```python
from build123d import *

# Parameters (mm, degrees)
EXTRUDE_1_DEPTH     = 50
SKETCH_4_W          = 44
SKETCH_4_H          = 13
CUT_EXTRUDE_2_DEPTH = 20
CUT_EXTRUDE_3_DEPTH = 88.252507127
SKETCH_6_R          = 11.05
SKETCH_6_R_2        = 1.6
CUT_EXTRUDE_4_DEPTH = 88.183714076


with BuildPart() as part:
    # 草图1 → 凸台-拉伸1 (new body)
    with BuildSketch(Plane(origin=(0, 0, 0), x_dir=(0, 0, -1), z_dir=(1, 0, 0))):
        Polygon((3, 0), (0, 0), (0, -51), (53, -51), (53, -48), (16, -48), (3, -28), align=None)
    extrude(amount=EXTRUDE_1_DEPTH)

    # 草图4 → 切除-拉伸2 (cut)
    with BuildSketch(Plane(origin=(0, -48, 0), x_dir=(1, 0, 0), z_dir=(0, 1, 0))):
        with Locations((25, 9.5)):
            Rectangle(SKETCH_4_W, SKETCH_4_H)
    extrude(amount=CUT_EXTRUDE_2_DEPTH, mode=Mode.SUBTRACT)

    # 草图5 → 切除-拉伸3 (cut, through all)
    with BuildSketch(Plane(origin=(0, -48, 0), x_dir=(1, 0, 0), z_dir=(0, 1, 0))):
        with BuildLine():
            Line((12.1, 42), (12.1, 12))
            ThreePointArc((12.1, 12), (10, 9.9), (7.9, 12))
            Line((7.9, 12), (7.9, 42))
            ThreePointArc((7.9, 42), (10, 44.1), (12.1, 42))
        make_face()
        with BuildLine():
            Line((37.9, 42), (37.9, 12))
            ThreePointArc((37.9, 12), (40, 9.9), (42.1, 12))
            Line((42.1, 12), (42.1, 42))
            ThreePointArc((42.1, 42), (40, 44.1), (37.9, 42))
        make_face()
        Polygon((50, 53), (45, 53), (50, 48), align=None)
        Polygon((5, 53), (0, 48), (0, 53), align=None)
    extrude(amount=-CUT_EXTRUDE_3_DEPTH, mode=Mode.SUBTRACT)

    # 草图6 → 切除-拉伸4 (cut, through all)
    with BuildSketch(Plane(origin=(0, 0, -3), x_dir=(-1, 0, 0), z_dir=(0, 0, -1))):
        with Locations(Location((-25, -21, 0), (0, 0, 90))):
            Circle(SKETCH_6_R)
        with Locations(Location((-40.5, -5.5, 0), (0, 0, 90))):
            Circle(SKETCH_6_R_2)
        with Locations(Location((-9.5, -5.5, 0), (0, 0, 90))):
            Circle(SKETCH_6_R_2)
        with Locations(Location((-9.5, -36.5, 0), (0, 0, 90))):
            Circle(SKETCH_6_R_2)
        with Locations(Location((-40.5, -36.5, 0), (0, 0, 90))):
            Circle(SKETCH_6_R_2)
        Polygon((-50, 0), (-50, -5), (-45, 0), align=None)
        Polygon((0, -5), (-5, 0), (0, 0), align=None)
    extrude(amount=-CUT_EXTRUDE_4_DEPTH, mode=Mode.SUBTRACT)


solid = part.part
```
The model under review builds one solid part; all positions refer to its coordinate system, in mm. A direction names the side the tool comes from. Round coordinates to 2 decimals unless told otherwise and drop trailing zeros. Write each loop counter-clockwise with the first axis right and the second up, starting at its lowest first coordinate (ties: lowest second). Pieces come first, ordered by that corner, then holes. Notation, with made-up numbers: (-3, -14.5) - (11, -14.5) arc R25 cw to (11, 14.5) - close; hole circle Ø9 at (-20, 77.25). An arc over 180 degrees is marked (long way). Use one line per item in the form item = value.
Q1. Insertion check: pin 1 Ø5 at (x, y) = (40.5, -36.5) entering from -Z; pin 2 Ø4 at (x, z) = (41, -6.5) entering from +Y; pin 3 Ø14.5 at (y, z) = (-34.5, -7.5) entering from +X. Each pin has a flat end and moves straight along its axis. Give the tip position at first contact, or say it passes through.
Answer key:
pin_1 = -3
pin_2 = -48
pin_3 = 50
Q2. Consider section C-C (z = -34.5). State the section outline as (x, y) points.
Answer key:
outline = (0, -51) - (7.9, -51) - (7.9, -48) - (0, -48) - close; (12.1, -51) - (37.9, -51) - (37.9, -48) - (12.1, -48) - close; (42.1, -51) - (50, -51) - (50, -48) - (42.1, -48) - close
Q3. Tool access review of faces 5 (the flat face through (3, -40, -8)), 6 (the flat face through (37.9, -49, -27)), 7 (the flat face through (50, -42, -11)): name each direction out of +Z, -Z, +X, -X, +Y, -Y from which nothing blocks a thin tool from reaching the whole face with its end or side.
Answer key:
face_5 = -Z, +Y
face_6 = +Y, -Y
face_7 = +Z, -Z, +X, +Y, -Y
Q4. Draft analysis for pull direction X (two halves, no side actions). For faces 1 (the flat face through (47, -49, -51)), 2 (the flat face through (36, -24, -3)), 3 (the flat face through (47, -40, -8)), 4 (the flat face through (0, -42, -11)), state which applies: +X half, -X half, draft (parallel to the pull), parting line (faces both ways), or undercut.
Answer key:
face_1 = +X half
face_2 = undercut
face_3 = undercut
face_4 = -X half
Q5. For line 1 (X direction, y = -36.5, z = -1.3); line 2 (X direction, y = -21, z = -0.7); line 3 (Y direction, x = 40, z = -2), list the stretches that pass through material, from the lowest coordinate up. Write a range as [from, to].
Answer key:
line_1 = [0, 7.9], [11.1, 38.9], [42.1, 50]
line_2 = [0, 13.95], [36.05, 50]
line_3 = [-51, -38.02], [-34.98, -7.02], [-3.98, 0]
Q6. Consider section D-D (x = 40.5). State the section outline as (y, z) points, and give its area (3 significant figures).
Answer key:
outline = (-51, -53) - (-48, -53) - (-48, -44.04) - (-51, -44.04) - close; (-51, -9.96) - (-48, -9.96) - (-48, -3) - (-38.1, -3) - (-38.1, 0) - (-51, 0) - close; (-34.9, -3) - (-7.1, -3) - (-7.1, 0) - (-34.9, 0) - close; (-3.9, -3) - (0, -3) - (0, 0) - (-3.9, 0) - close
area = 182 mm2
Q7. Consider section A-A (x = 25). State the section outline as (y, z) points.
Answer key:
outline = (-51, -53) - (-48, -53) - (-48, -3) - (-32.05, -3) - (-32.05, 0) - (-51, 0) - close; (-9.95, -3) - (0, -3) - (0, 0) - (-9.95, 0) - close
Q8. Consider section B-B (y = -21). State the section outline as (x, z) points.
Answer key:
outline = (0, -3) - (13.95, -3) - (13.95, 0) - (0, 0) - close; (36.05, -3) - (50, -3) - (50, 0) - (36.05, 0) - close
